Here's the drawing with two shaded views (mm, measured from the low corner). I have some questions. Give positions to 0.01 mm unless a question says otherwise; leave off trailing zeros. Write each loop counter-clockwise with the first axis right and the second up, starting at its lowest first coordinate (ties: lowest second). Pieces come first, ordered by that corner, then holes. Notation, with made-up numbers: (-27, -30) -> (-14, -30) arc R21 ccw to (-14, 4) -> close; hole circle Ø6 at (49, 82). An arc over 180 degrees is marked (long way). One line per question, with ' | ' between items.
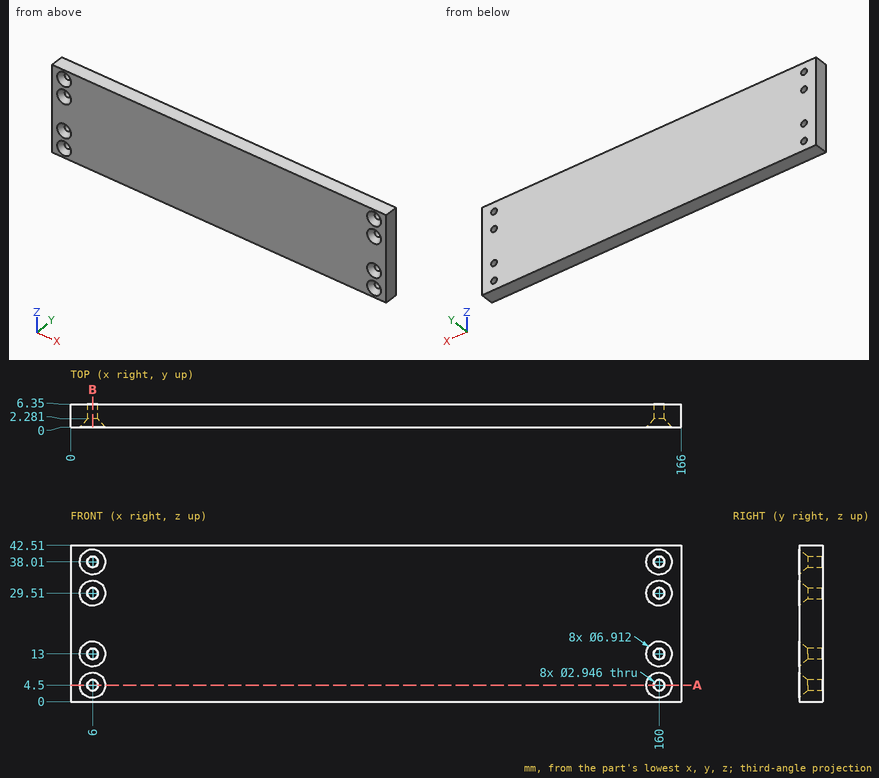
Q1. If I drill on line 1 along X through (y, z) = (3.85, 13); line 2 along Z through (x, y) = (160, 4.3); line 3 along X through (y, z) = (4.75, 29), over which ranges is the centre line in solid material (lowest first)?
Answer below:
line 1: x = 0 to 4.53, 7.47 to 158.53, 161.47 to 166 | line 2: z = 0 to 3.03, 5.97 to 11.53, 14.47 to 28.04, 30.98 to 36.54, 39.48 to 42.51 | line 3: x = 0 to 4.62, 7.38 to 158.62, 161.38 to 166
Q2. Imagine slicing it at A-A on z = 4.5. Please give me the cut outline in (x, y).
Answer below:
outline: (0, 0) -> (2.54, 0) -> (4.53, 2.28) -> (4.53, 6.35) -> (0, 6.35) -> close; (7.47, 2.28) -> (9.46, 0) -> (156.54, 0) -> (158.53, 2.28) -> (158.53, 6.35) -> (7.47, 6.35) -> close; (161.47, 2.28) -> (163.46, 0) -> (166, 0) -> (166, 6.35) -> (161.47, 6.35) -> close
Q3. Will these pins go through, and if not, where does the flat tip stop? pin 1 (4.5 mm diameter, centred on x = 160, z = 38.01, fed in from -Y); pin 2 (3.5 mm diameter, centred on x = 160, z = 29.51, fed in from -Y); pin 3 (2.5 mm diameter, centred on x = 6, z = 38.01, fed in from +Y).
Answer below:
pin 1: stops at y = 1.39 | pin 2: stops at y = 1.96 | pin 3: passes through
Q4. Imagine slicing it at B-B on x = 6. Please give me the cut outline in (y, z).
Answer below:
outline: (0, 0) -> (6.35, 0) -> (6.35, 3.03) -> (2.28, 3.03) -> (0, 1.04) -> close; (0, 7.96) -> (2.28, 5.97) -> (6.35, 5.97) -> (6.35, 11.53) -> (2.28, 11.53) -> (0, 9.54) -> close; (0, 16.46) -> (2.28, 14.47) -> (6.35, 14.47) -> (6.35, 28.04) -> (2.28, 28.04) -> (0, 26.05) -> close; (0, 32.97) -> (2.28, 30.98) -> (6.35, 30.98) -> (6.35, 36.54) -> (2.28, 36.54) -> (0, 34.55) -> close; (0, 41.47) -> (2.28, 39.48) -> (6.35, 39.48) -> (6.35, 42.51) -> (0, 42.51) -> close
